Input: dimensioned drawing with shaded views. Units: mm. Origin: part minimum x, y, z. A direction names the side the tool comes from. Round coordinates to 2 decimals unless told otherwise and drop trailing zeros. Loops run counter-clockwise (first coordinate to the right, second up) from the corner with the lowest first, then second, coordinate; pieces in that order, holes last. Notation, with made-up numbers: M 63,51.5 L 67,51.5 A22 ccw 67,74.5 Z; hole C 10,-38.75 d2. An arc over 180 degrees is marked long. Answer as CSV lines item,"result". Start each with the question number.
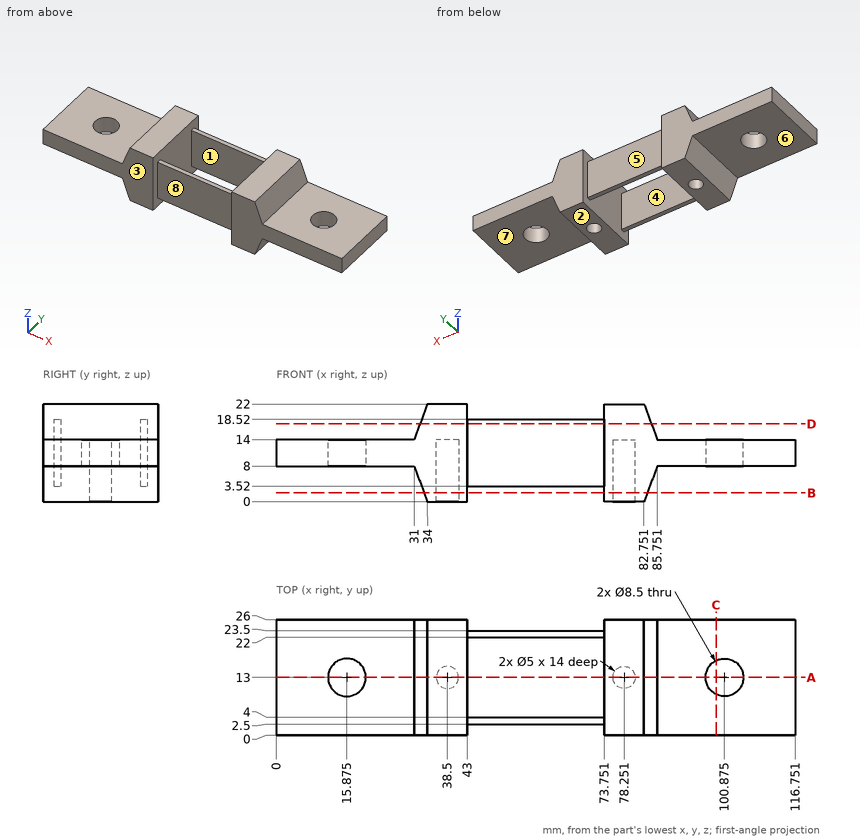
1) Section C-C, the plane x = 99. Return loops of the section in (y, z), and give its area (3 significant figures).
2) Ray query, line 1 along X through (y, z) = (12, 6); line 2 along Y through (x, z) = (68.5, 5); line 3 along X through (y, z) = (15.25, 11.25). Return the intervals inside material, ascending.
3) Contact query for flat-ended pins moving along their axis: pin 1 Ø8 at (x, y) = (101.5, 18) entering from +Z; pin 2 Ø4 at (x, y) = (38.5, 13) entering from -Z; pin 3 Ø12 at (x, z) = (51, 8) entering from +Y. Output: stop coordinate, or through.
4) Section B-B, the plane z = 2. Return loops of the section in (x, y).
5) Mould query, pull axis Y, two halves, no side actions, for the marked faces 1, 2, 3 and 4. Classes: pulls with the +Y half, pulls with the -Y half, needs draft (parallel to the pull), parting line crosses it, or undercut.
6) Section D-D, the plane z = 17.5. Return loops of the section in (x, y).
7) Access query for the marked faces 5, 6, 7 and 8. Directions: +Z, -Z, +X, -X, +Y, -Y. A direction counts if a zero-diameter tool reaches every point of the face in a straight line with its end or side. Return the directions, or none.
8) Section A-A, the plane y = 13. Give the number of separate pieces and of enclosed holes in the cut face, and give its area (3 significant figures).
Findings below:
1,outline,"M 0,8 L 9.19,8 L 9.19,14 L 0,14 Z; M 16.81,8 L 26,8 L 26,14 L 16.81,14 Z"
1,area,"110 mm²"
2,line 1,"31.75 to 36.21, 40.79 to 43, 73.75 to 75.96, 80.54 to 85"
2,line 2,"2.5 to 4, 22 to 23.5"
2,line 3,"0 to 12.27, 19.48 to 37.41, 39.59 to 43, 73.75 to 77.16, 79.34 to 97.27, 104.48 to 116.75"
3,pin 1,"z = 14"
3,pin 2,"z = 14"
3,pin 3,"y = 23.5"
4,outline,"M 33.25,0 L 43,0 L 43,26 L 33.25,26 Z; M 73.75,0 L 83.5,0 L 83.5,26 L 73.75,26 Z; hole C 38.5,13 d5; hole C 78.25,13 d5"
5,face 1,"undercut"
5,face 2,"needs draft"
5,face 3,"pulls with the -Y half"
5,face 4,"undercut"
6,outline,"M 32.31,0 L 43,0 L 43,2.5 L 73.75,2.5 L 73.75,0 L 84.44,0 L 84.44,26 L 73.75,26 L 73.75,23.5 L 43,23.5 L 43,26 L 32.31,26 Z; hole M 43,4 L 73.75,4 L 73.75,22 L 43,22 Z"
7,face 5,"+Z, -Z, +Y"
7,face 6,"-Z, -X, +Y, -Y"
7,face 7,"-Z, +X, +Y, -Y"
7,face 8,"+Z, -Z, -Y"
8,separate pieces,"4"
8,enclosed holes,"0"
8,area,"610 mm²"
